Source: CAD feature listing. Evaluate the final solid. Frame: model axes, mm. Face numbers are marked on the shaded views. A direction names the side the tool comes from. Give positions to 0.01 mm unless a question says otherwise; leave off trailing zeros. Order: outer loops, then holes, each group sorted by start corner. A loop starts at its lowest first (then second) coordinate and runs counter-clockwise, first axis right, second up. Notation, with made-up numbers: (16.5, 56) -> (22.5, 56) arc R21 cw to (22.5, 64) -> close; hole circle Ø9 at (25.25, 0.5). An arc over 180 degrees is marked (long way). Use one line per item in the form item = value. Start each with the question number.
from build123d import *

# Parameters (mm, degrees)
SKETCH_1_W                      = 35
SKETCH_1_H                      = 8
EXTRUDE_2_DEPTH                 = 10
CUT_EXTRUDE_4_DEPTH             = 3
SKETCH_11_W                     = 35
SKETCH_11_H                     = 8
CUT_EXTRUDE_5_DEPTH             = 7
SKETCH_14_W                     = 2
SKETCH_14_H                     = 8
EXTRUDE_7_DEPTH                 = 10
CUT_EXTRUDE_6_DEPTH             = 38.815340802
CUT_EXTRUDE_6_DEPTH_BACK        = 3
SKETCH_12_R                     = 1.5
EXTRUDE_10_DEPTH                = 8
CUT_EXTRUDE_8_REACH             = 42.608
SKETCH_31_W                     = 26
SKETCH_31_H                     = 4
CUT_EXTRUDE_8_DIRECTION_2_DEPTH = 41.607881008


with BuildPart() as part:
    # 草图1 → 凸台-拉伸2 (new body)
    with BuildSketch(Plane.XY):
        Polygon((0, 4), (-3, 6), (-3, 2), (0, 2), align=None)
        Polygon((0, 6), (0, 4), (0, 0), (0, -2), (3, -2), (3, 6), align=None)
        Polygon((0, 2), (-3, 2), (-3, -2), (0, 0), align=None)
        with Locations((20.5, 2)):
            Rectangle(SKETCH_1_W, SKETCH_1_H)
    extrude(amount=EXTRUDE_2_DEPTH)

    # 草图1<4> → 切除-拉伸4 (cut)
    with BuildSketch(Plane.XY):
        Polygon((0, 4), (-3, 6), (-3, 2), (0, 2), align=None)
        Polygon((0, 2), (-3, 2), (-3, -2), (0, 0), align=None)
    extrude(amount=CUT_EXTRUDE_4_DEPTH, mode=Mode.SUBTRACT)

    # 草图11 → 切除-拉伸5 (cut)
    with BuildSketch(Plane.XY.offset(10)):
        with Locations((20.5, 2)):
            Rectangle(SKETCH_11_W, SKETCH_11_H)
    extrude(amount=-CUT_EXTRUDE_5_DEPTH, mode=Mode.SUBTRACT)

    # 草图14 → 凸台-拉伸7 (add)
    with BuildSketch(Plane.XY.offset(3)):
        with Locations((37, 2)):
            Rectangle(SKETCH_14_W, SKETCH_14_H)
        with Locations((9, 2)):
            Rectangle(SKETCH_14_W, SKETCH_14_H)
    extrude(amount=EXTRUDE_7_DEPTH)

    # 草图12 → 切除-拉伸6 (cut, two sides: drawn at the far end of the back side and taken through both)
    with BuildSketch(Plane(origin=(3, 0, 0), x_dir=(0, 0, -1), z_dir=(1, 0, 0)).offset(-CUT_EXTRUDE_6_DEPTH_BACK)):
        with Locations((-6.5, 2)):
            Circle(SKETCH_12_R)
    extrude(amount=CUT_EXTRUDE_6_DEPTH + CUT_EXTRUDE_6_DEPTH_BACK, mode=Mode.SUBTRACT)

    # 草图30 → 凸台-拉伸10 (add)
    with BuildSketch(Plane(origin=(0, 6, 0), x_dir=(1, 0, 0), z_dir=(0, 1, 0))):
        with BuildLine():
            Line((10, -11), (10, -13))
            ThreePointArc((10, -13), (23, -11.574738582), (36, -13))
            Line((36, -13), (36, -11))
            ThreePointArc((36, -11), (23, -9.574738582), (10, -11))
        make_face()
    extrude(amount=-EXTRUDE_10_DEPTH)

    # 草图31 → 切除-拉伸8 (cut, up to next)
    with BuildSketch(Plane.XY.offset(13), mode=Mode.PRIVATE) as cut_extrude_8_sk1:
        with Locations((23, 2)):
            Rectangle(SKETCH_31_W, SKETCH_31_H)
    cut_extrude_8_tool1 = extrude(cut_extrude_8_sk1.sketch, amount=-CUT_EXTRUDE_8_REACH, mode=Mode.PRIVATE) & part.part
    add(cut_extrude_8_tool1.solids().sort_by_distance((23, 2, 13))[0], mode=Mode.SUBTRACT)

    # 草图31 → 切除-拉伸8 direction 2 (cut)
    with BuildSketch(Plane.XY.offset(13)):
        with Locations((23, 2)):
            Rectangle(SKETCH_31_W, SKETCH_31_H)
    extrude(amount=CUT_EXTRUDE_8_DIRECTION_2_DEPTH, mode=Mode.SUBTRACT)


solid = part.part
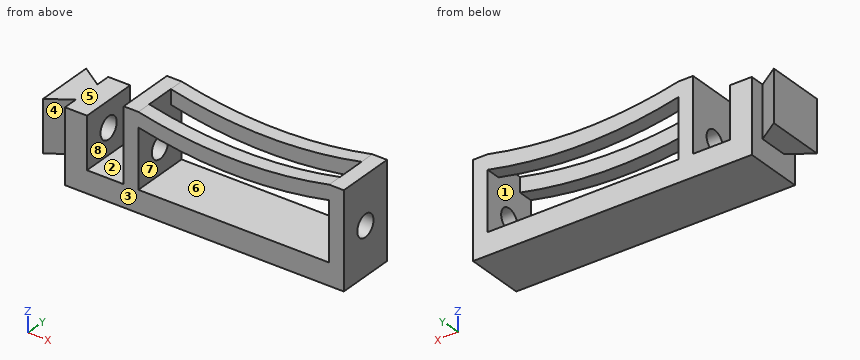
1) Cut plane A-A, the plane y = 5.5. Return the cut outline in (x, z), plus the area to 3 significant figures.
2) Pin query (flat end, axial travel): pin 1 (1 mm diameter, centred on x = 2.5, y = 0, fed in from +Z); pin 2 (2.5 mm diameter, centred on y = 2, z = 6.5, fed in from +X); pin 3 (2.5 mm diameter, centred on x = 17, y = 0, fed in from +Z). Return the tip coordinate at first contact, or that it passes through.
3) Reachability of the marked faces 4, 5, 6, 7 and 8 from +Z, -Z, +X, -X, +Y, -Y: full face, straight path, thin tool, end or side. Return the list, or none.
4) Cut plane C-C, the plane y = 2. Return the cut outline in (x, z), plus the area to 3 significant figures.
5) Cut plane D-D, the plane z = 6.5. Return the cut outline in (x, y).
6) Cut plane B-B, the plane z = 9. Return the cut outline in (x, y).
7) Draft query along Z for the marked faces 1, 2 and 3. Return one class per face: +Z half, -Z half, draft (parallel to the pull), parting line (faces both ways), or undercut.
8) Material intervals for probe 1 along X at (y, z) = (2.5, 9.5); probe 2 along Z at (x, y) = (8.75, 2); probe 3 along Y at (x, z) = (9.25, 6.5), sorted ascending.
Output values:
q1.outline = (-3, 3) -> (-2.25, 3) -> (-2.25, 10) -> (-3, 10) -> close; (0, 0) -> (38, 0) -> (38, 13) -> (36, 13) arc R60 cw to (10, 13) -> (8, 13) -> (8, 3) -> (3, 3) -> (3, 10) -> (0, 10) -> close; hole (10, 3) -> (36, 3) -> (36, 11) arc R60 cw to (10, 11) -> close
q1.area = 232 mm^2
q2.pin_1 = 10
q2.pin_2 = 0
q2.pin_3 = 12.01
q3.face_4 = +Z, -Z, -Y
q3.face_5 = +Z, -X, +Y, -Y
q3.face_6 = +Y, -Y
q3.face_7 = none
q3.face_8 = +Z, +Y, -Y
q4.outline = (-3, 3) -> (0, 3) -> (0, 0) -> (38, 0) -> (38, 5) -> (36, 5) -> (36, 3) -> (10, 3) -> (10, 5) -> (8, 5) -> (8, 3) -> (3, 3) -> (3, 5) -> (0, 5) -> (0, 8) -> (3, 8) -> (3, 10) -> (-3, 10) -> close; (8, 8) -> (10, 8) -> (10, 13) -> (8, 13) -> close; (36, 8) -> (38, 8) -> (38, 13) -> (36, 13) -> close
q4.area = 175 mm^2
q5.outline = (-3, -2) -> (0, 0) -> (0, -2) -> (3, -2) -> (3, 0.5) -> (0, 0.5) -> (0, 3.5) -> (3, 3.5) -> (3, 6) -> (0, 6) -> (0, 4) -> (-3, 6) -> close; (8, -2) -> (10, -2) -> (10, 0.5) -> (8, 0.5) -> close; (8, 3.5) -> (10, 3.5) -> (10, 6) -> (8, 6) -> close; (36, -2) -> (38, -2) -> (38, 0.5) -> (36, 0.5) -> close; (36, 3.5) -> (38, 3.5) -> (38, 6) -> (36, 6) -> close
q6.outline = (-3, -2) -> (0, 0) -> (0, -2) -> (3, -2) -> (3, 6) -> (0, 6) -> (0, 4) -> (-3, 6) -> close; (8, -2) -> (10, -2) -> (10, 6) -> (8, 6) -> close; (36, -2) -> (38, -2) -> (38, 6) -> (36, 6) -> close
q7.face_1 = undercut
q7.face_2 = +Z half
q7.face_3 = draft
q8.probe_1 = -3 to 3, 8 to 10, 36 to 38
q8.probe_2 = 0 to 5, 8 to 13
q8.probe_3 = -2 to 0.5, 3.5 to 6
